Autodesk Fusion 360 part; units mm, degrees
sketch "Sketch1" plane through (0, 0, 0) normal (0, 1, 0) x (1, 0, 0)
  line L0 (0, 6.6056) -> (0, 28)
  line L1 (2, 30) -> (16.263, 30)
  line L2 (17.9271, 26.8906) -> (3.6641, 5.4962)
  arc A0 (2, 30) -> (0, 28) centre (2, 28) ccw
  arc A1 (0, 6.6056) -> (3.6641, 5.4962) centre (2, 6.6056) ccw
  arc A2 (17.9271, 26.8906) -> (16.263, 30) centre (16.263, 28) ccw
  circle A3 centre (2, 28) radius 1
  circle A4 centre (16.263, 28) radius 1
  circle A5 centre (2, 6.6056) radius 1
  point P0 (0, 30)
  point P1 (20, 30)
  dimension "d1" = 20
  dimension "d2" = 30
  dimension "d3" = 2
  dimension "d4" = 2
  dimension "d5" = 2
  dimension "d6" = 2
  dimension "d7" = 2
  dimension "d8" = 2
extrude "Extrude1" add sketch "Sketch1" along normal blind 2
CAD build for the part. Positions are in the model's coordinates, mm. Round coordinates to 2 decimals unless told otherwise and drop trailing zeros. Order: outer loops, then holes, each group sorted by start corner. A loop starts at its lowest first (then second) coordinate and runs counter-clockwise, first axis right, second up. Notation, with made-up numbers: (-17.75, 9) - (1.25, 9) arc R18 ccw to (1.25, 19) - close; hole circle Ø2 at (82.25, 12). An arc over 180 degrees is marked (long way). Use CSV: the item, a comma, the result in double quotes. Start each with the question number.
1) Saw through at B-B (x = 12). List the corners of the cut face in (y, z), and give its area (3 significant figures).
2) Pin check, flat tips, straight feed: pin 1 Ø1.8 at (x, z) = (2, -6.61) entering from +Y; pin 2 Ø3 at (x, z) = (16.263, -28) entering from +Y. Stop position of each tip, or through.
3) Saw through at C-C (z = -15). List the corners of the cut face in (x, y), and give its area (3 significant figures).
4) Two-plate mould, pull along X, no slides. Class faces 1 (the cylindrical face through (15.53, 0.99, -27.32)), 2 (the flat face through (0, 1, -17)), 3 (the flat face through (7, 0, -20)): pulls with the +X half, pulls with the -X half, needs draft (parallel to the pull), parting line crosses it, or undercut.
5) Saw through at A-A (y = 0.3). List the corners of the cut face in (x, z).
6) Wall check: L1, parallel to X at y = 1.05, z = -28; L2, parallel to Z at x = 2, y = 0.6; L3, parallel to Z at x = 2.75, y = 0.8. Give the ranges that are in metal, low to high. Write a range as [from, to].
Values follow:
1,outline,"(0, -30) - (2, -30) - (2, -18) - (0, -18) - close"
1,area,"24.0 mm2"
2,pin 1,"passes through"
2,pin 2,"stops at y = 2"
3,outline,"(0, 0) - (10, 0) - (10, 2) - (0, 2) - close"
3,area,"20.0 mm2"
4,face 1,"undercut"
4,face 2,"pulls with the -X half"
4,face 3,"needs draft"
5,outline,"(0, -28) arc R2 ccw to (2, -30) - (16.26, -30) arc R2 ccw to (17.93, -26.89) - (3.66, -5.5) arc R2 ccw to (0, -6.61) - close; hole circle Ø2 at (2, -28); hole circle Ø2 at (2, -6.61); hole circle Ø2 at (16.26, -28)"
6,L1,"x = [0, 1], [3, 15.26], [17.26, 18.26]"
6,L2,"z = [-30, -29], [-27, -7.61], [-5.61, -4.61]"
6,L3,"z = [-30, -28.66], [-27.34, -7.27], [-5.94, -4.75]"
